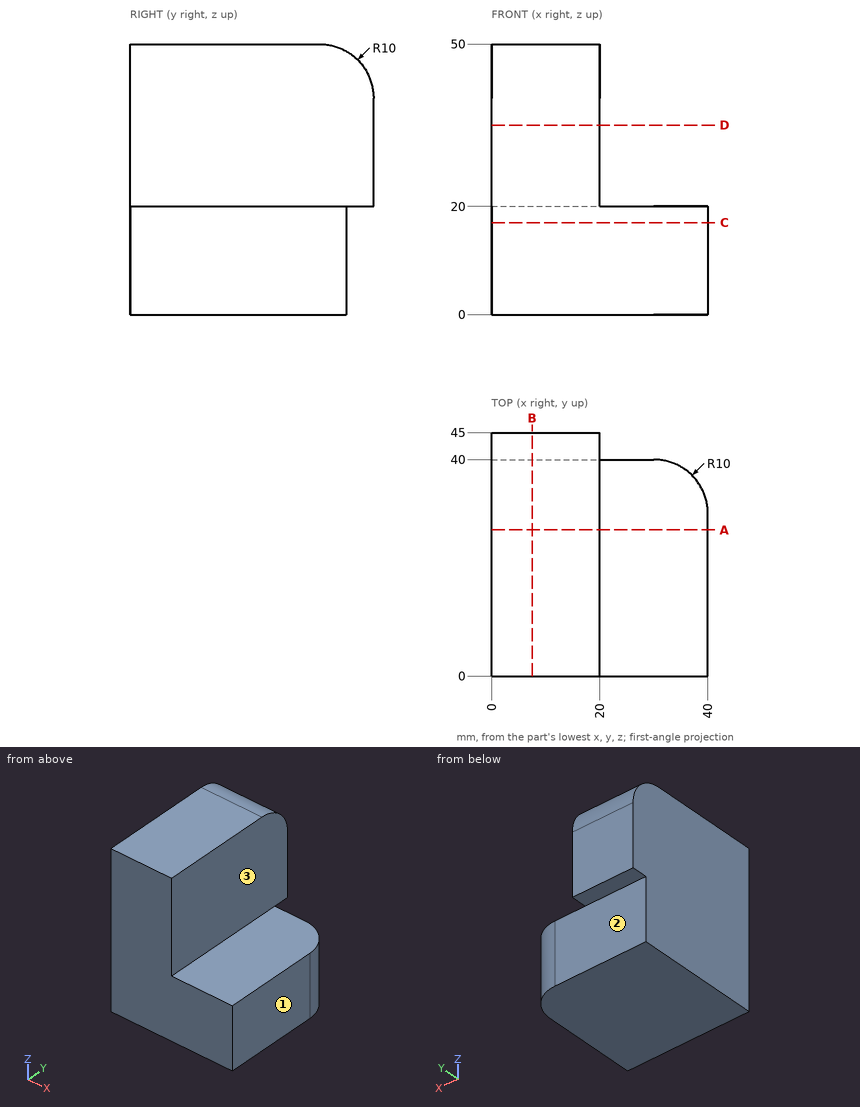
The figure shows three views and two pictorial views of one solid part (mm, origin at its lowest corner). Answer the questions. A direction names the side the tool comes from. Give positions to 0.01 mm unless a question says otherwise; leave off trailing zeros. Loops run counter-clockwise (first coordinate to the right, second up) from the corner with the lowest first, then second, coordinate; pieces in that order, holes last. Notation, with made-up numbers: (28.5, 25.5) -> (61.5, 25.5) arc R20 ccw to (61.5, 57.5) -> close; hole circle Ø2 at (23.25, 57). An arc over 180 degrees is marked (long way). Put each result on its own line as item: value. Start each with the question number.
Item 1: The part is cut by section A-A (y = 27). Give the vertices of the cut face in (x, z).
Item 2: Which of the six approach directions +Z, -Z, +X, -X, +Y, -Y give full straight-line access (tool end or side, diameter ignored) to the marked faces 1, 2 and 3?
Item 3: Each of these flat-tipped pins is pushed along its axis until it touches: P1, Ø2.5, axis at x = 6, y = 42.5, coming from the -Z side; P2, Ø1.5, axis at y = 7, z = 41, coming from the +X side; P3, Ø10, axis at x = 8, z = 5.5, coming from the +Y side. Where does it stop, or does it pass through?
Item 4: The part is cut by section C-C (z = 17). Give the vertices of the cut face in (x, y).
Item 5: The part is cut by section B-B (x = 7.5). Give the vertices of the cut face in (y, z).
Item 6: Find the intervals of material crossed by L1, parallel to X at y = 41.5, z = 36.5; L2, parallel to Y at x = 16, z = 13.5, in increasing order. Write a range as [from, to].
Item 7: The part is cut by section D-D (z = 35). Give the vertices of the cut face in (x, y).
Answers below:
1. outline: (0, 0) -> (40, 0) -> (40, 20) -> (20, 20) -> (20, 50) -> (0, 50) -> close
2. face 1: +Z, -Z, +X, +Y, -Y
2. face 2: -Z, +X, -X, +Y
2. face 3: +Z, +X, +Y, -Y
3. P1: z = 20
3. P2: x = 20
3. P3: y = 40
4. outline: (0, 0) -> (40, 0) -> (40, 30) arc R10 ccw to (30, 40) -> (0, 40) -> close
5. outline: (0, 0) -> (40, 0) -> (40, 20) -> (45, 20) -> (45, 40) arc R10 ccw to (35, 50) -> (0, 50) -> close
6. L1: [0, 20]
6. L2: [0, 40]
7. outline: (0, 0) -> (20, 0) -> (20, 45) -> (0, 45) -> close
